Can you work these out from the model? Positions are in its coordinate system, mm. Face numbers are marked on the shaded views. A direction names the side the tool comes from. Give positions to 0.01 mm unless a question says otherwise; leave off trailing zeros. Loops run counter-clockwise (first coordinate to the right, second up) from the corner with the lowest first, then second, coordinate; pieces in that order, holes last.
from build123d import *

# Parameters (mm, degrees)
EXTRUDE_1_DEPTH          = 35
CUT_EXTRUDE_1_DEPTH      = 30
SKETCH_3_R               = 10
CUT_EXTRUDE_2_DEPTH      = 1
CUT_EXTRUDE_2_DEPTH_BACK = 71
CUT_EXTRUDE_3_REACH      = 7
SKETCH_4_R               = 15
EXTRUDE_2_DEPTH          = 5
HOLE_WIZARD_M4_1_D       = 3.3
HOLE_WIZARD_M4_1_DEPTH   = 5
HOLE_WIZARD_M4_2_D       = 3.3
HOLE_WIZARD_M4_2_DEPTH   = 5
HOLE_WIZARD_M4_3_D       = 3.3


with BuildPart() as part:
    # 스케치1 → 보스-돌출1 (new body)
    with BuildSketch(Plane(origin=(0, 0, 0), x_dir=(1, 0, 0), z_dir=(0, 1, 0))):
        with BuildLine():
            Line((-26, 35), (26, 35))
            ThreePointArc((26, 35), (61, 0), (26, -35))
            Line((26, -35), (-26, -35))
            ThreePointArc((-26, -35), (-61, 0), (-26, 35))
        make_face()
    extrude(amount=EXTRUDE_1_DEPTH)

    # 스케치2 → 컷-돌출1 (cut)
    with BuildSketch(Plane(origin=(0, 35, 0), x_dir=(1, 0, 0), z_dir=(0, 1, 0))):
        with BuildLine():
            Line((26, 30), (-26, 30))
            ThreePointArc((-26, 30), (-56, 0), (-26, -30))
            Line((-26, -30), (26, -30))
            ThreePointArc((26, -30), (56, 0), (26, 30))
        make_face()
    extrude(amount=-CUT_EXTRUDE_1_DEPTH, mode=Mode.SUBTRACT)

    # 스케치3 → 컷-돌출2 (cut, two sides)
    with BuildSketch(Plane.XY.offset(35)) as cut_extrude_2_sk:
        with Locations((0, 35)):
            Circle(SKETCH_3_R)
    extrude(amount=CUT_EXTRUDE_2_DEPTH, mode=Mode.SUBTRACT)
    extrude(cut_extrude_2_sk.sketch, amount=-CUT_EXTRUDE_2_DEPTH_BACK, mode=Mode.SUBTRACT)

    # 스케치4 → 컷-돌출3 (cut, up to next)
    with BuildSketch(Plane(origin=(0, 5, 0), x_dir=(1, 0, 0), z_dir=(0, 1, 0)), mode=Mode.PRIVATE) as cut_extrude_3_sk1:
        Circle(SKETCH_4_R)
    cut_extrude_3_tool1 = extrude(cut_extrude_3_sk1.sketch, amount=-CUT_EXTRUDE_3_REACH, mode=Mode.PRIVATE) & part.part
    add(cut_extrude_3_tool1.solids().sort_by_distance((0, 5, 0))[0], mode=Mode.SUBTRACT)

    # 스케치5 → 보스-돌출2 (add)
    with BuildSketch(Plane(origin=(0, 35, 0), x_dir=(1, 0, 0), z_dir=(0, 1, 0))):
        with BuildLine():
            Line((-10, 32), (-26, 32))
            ThreePointArc((-26, 32), (-58, 0), (-26, -32))
            Line((-26, -32), (-10, -32))
            Line((-10, -32), (-10, -30))
            Line((-10, -30), (-26, -30))
            ThreePointArc((-26, -30), (-56, 0), (-26, 30))
            Line((-26, 30), (-10, 30))
            Line((-10, 30), (-10, 32))
        make_face()
        with BuildLine():
            Line((10, -32), (26, -32))
            ThreePointArc((26, -32), (58, 0), (26, 32))
            Line((26, 32), (10, 32))
            Line((10, 32), (10, 30))
            Line((10, 30), (26, 30))
            ThreePointArc((26, 30), (56, 0), (26, -30))
            Line((26, -30), (10, -30))
            Line((10, -30), (10, -32))
        make_face()
    extrude(amount=EXTRUDE_2_DEPTH)

    # M4 나사 구멍1
    with Locations(Plane.XY.offset(35)):
        with Locations((-10.606601718, 24.393398282), (10.606601718, 24.393398282)):
            Hole(HOLE_WIZARD_M4_1_D / 2, depth=HOLE_WIZARD_M4_1_DEPTH)

    # M4 나사 구멍2
    with Locations(Plane(origin=(0, 0, -35), x_dir=(-1, 0, 0), z_dir=(0, 0, -1))):
        with Locations((-10.606601718, 24.393398282), (10.606601718, 24.393398282)):
            Hole(HOLE_WIZARD_M4_2_D / 2, depth=HOLE_WIZARD_M4_2_DEPTH)

    # M4 나사 구멍3 (through all)
    with Locations(Plane(origin=(0, 5, 0), x_dir=(1, 0, 0), z_dir=(0, 1, 0))):
        with Locations((0, 22), (-20, 0), (50, 0), (0, -22)):
            Hole(HOLE_WIZARD_M4_3_D / 2)


solid = part.part
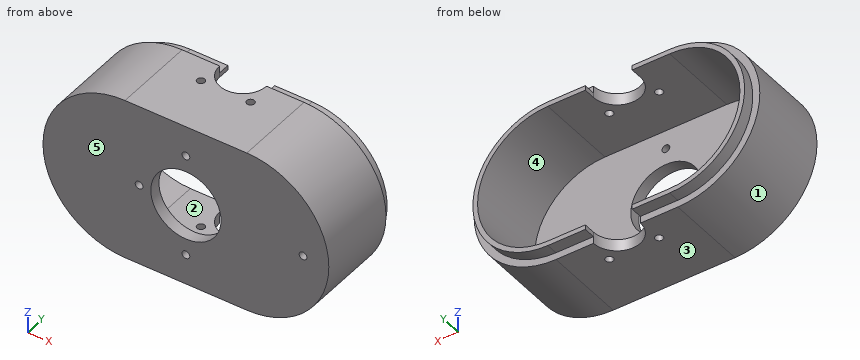
(1) Will these pins go through, and if not, where does the flat tip stop? P1, Ø1, axis at x = -30, y = 13, coming from the +Z side; P2, Ø4, axis at x = -20, z = 0, coming from the +Y side; P3, Ø5.5, axis at x = -18, y = 38, coming from the +Z side; P4, Ø2, axis at x = 0, z = 22, coming from the -Y side.
Returned:
P1: stops at z = 34.82
P2: stops at y = 5
P3: stops at z = 32
P4: passes through
(2) Suppose I cut it at B-B on y = 13. List the corners of the cut face in (x, z) for me.
Returned:
outline: (-26, -35) - (26, -35) arc R35 ccw to (26, 35) - (-26, 35) arc R35 ccw to start; hole (-26, -30) - (26, -30) arc R30 ccw to (26, 30) - (-26, 30) arc R30 ccw to start
(3) Suppose I cut it at D-D on x = -44. List the corners of the cut face in (y, z) for me.
Returned:
outline: (0, -30.02) - (35, -30.02) - (35, -26.46) - (40, -26.46) - (40, -24) - (5, -24) - (5, 24) - (40, 24) - (40, 26.46) - (35, 26.46) - (35, 30.02) - (0, 30.02) - close
(4) Please list where these lines run through material, in increasing order: probe 1 along Z at (x, y) = (0, 2.4); probe 2 along Z at (x, y) = (25.5, 31.5); probe 3 along X at (y, z) = (13, -0.5).
Returned:
probe 1: z = -35 to -23.65, -20.35 to -15, 15 to 20.35, 23.65 to 35
probe 2: z = -35 to -30, 30 to 35
probe 3: x = -61 to -56, 56 to 61
(5) Thinking about a two-plate mould opening in Z: for the marked faces 3, 4 and 5, which applies, pulls with the +Z half, pulls with the -Z half, needs draft (parallel to the pull), parting line crosses it, or undercut?
Returned:
face 3: pulls with the -Z half
face 4: undercut
face 5: needs draft
(6) Suppose I cut it at A-A on x = -20. List the corners of the cut face in (y, z) for me.
Returned:
outline: (0, -35) - (35, -35) - (35, -32) - (40, -32) - (40, -30) - (5, -30) - (5, -1.65) - (0, -1.65) - close; (0, 1.65) - (5, 1.65) - (5, 30) - (40, 30) - (40, 32) - (35, 32) - (35, 35) - (0, 35) - close
(7) Which directions (+Z, -Z, +X, -X, +Y, -Y) give clear straight access to the entire face, cutting with the end or side of a thin tool? Please do the marked faces 1 and 2.
Returned:
face 1: -X, +Y, -Y
face 2: +Y
(8) Suppose I cut it at C-C on z = -12. List the corners of the cut face in (x, y) for me.
Returned:
outline: (-58.88, 0) - (-9, 0) - (-9, 5) - (-53.5, 5) - (-53.5, 40) - (-55.66, 40) - (-55.66, 35) - (-58.88, 35) - close; (9, 0) - (58.88, 0) - (58.88, 35) - (55.66, 35) - (55.66, 40) - (53.5, 40) - (53.5, 5) - (9, 5) - close
